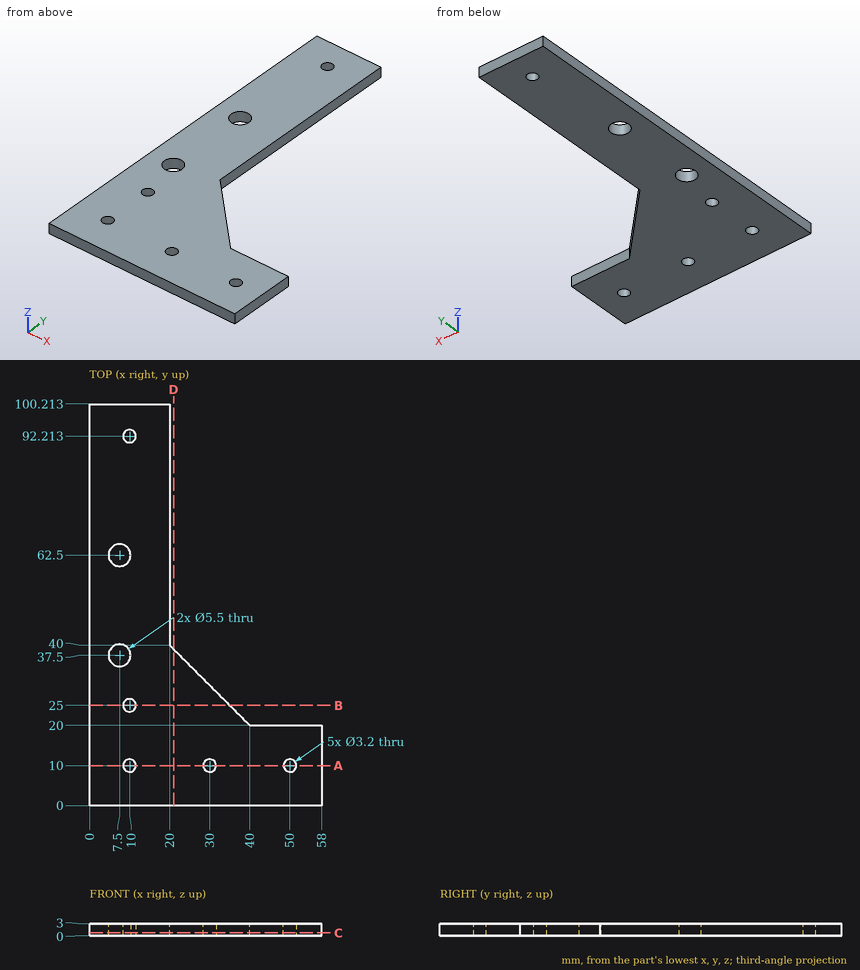
For this review, use the dimensioned drawing (mm, ordinates from the lowest corner) and the shaded views. Coordinates: 2 decimals unless noted, no trailing zeros. Order: outer loops, then holes, each group sorted by start corner. A loop starts at its lowest first (then second) coordinate and runs counter-clockwise, first axis right, second up. Notation, with made-up numbers: M 21,-33.5 L 70,-33.5 A24 ccw 70,4.5 Z; hole C 2.25,-16.75 d11. An arc over 180 degrees is marked long. Answer as a JSON object with one key per item and string values. Group by question number.
1) Wall thickness on L1, parallel to Y at x = 7.5, z = 1.8; L2, parallel to X at y = 75, z = 2.05; L3, parallel to X at y = 35, z = 2.4 (1 decimal): over which ranges is each line inside the solid? List them lowest first.
2) Add section B-B, the plane y = 25. Write out the cut boundary in (x, z).
3) Add section D-D, the plane x = 21. Write out the cut boundary in (y, z), then the cut area to 3 significant figures.
4) Add section A-A, the plane y = 10. Write out the cut boundary in (x, z), then the cut area to 3 significant figures.
5) For pin 1 (1.5 mm diameter, centred on y = 82, z = 1, fed in from +X); pin 2 (1.5 mm diameter, centred on x = 28.5, z = 1.5, fed in from +Y), all flat-tipped, find the tip position at first contact; note any pin that passes through.
6) Add section C-C, the plane z = 0.7. Write out the cut boundary in (x, y).
Computed values:
{
 "1": {"L1": "y = 0 to 34.75, 40.25 to 59.75, 65.25 to 100.21", "L2": "x = 0 to 20", "L3": "x = 0 to 6.4, 8.6 to 25"},
 "2": {"outline": "M 0,0 L 8.4,0 L 8.4,3 L 0,3 Z; M 11.6,0 L 35,0 L 35,3 L 11.6,3 Z"},
 "3": {"outline": "M 0,0 L 39,0 L 39,3 L 0,3 Z", "area": "117 mm^2"},
 "4": {"outline": "M 0,0 L 8.4,0 L 8.4,3 L 0,3 Z; M 11.6,0 L 28.4,0 L 28.4,3 L 11.6,3 Z; M 31.6,0 L 48.4,0 L 48.4,3 L 31.6,3 Z; M 51.6,0 L 58,0 L 58,3 L 51.6,3 Z", "area": "145 mm^2"},
 "5": {"pin 1": "stops at x = 20", "pin 2": "stops at y = 32.25"},
 "6": {"outline": "M 0,0 L 58,0 L 58,20 L 40,20 L 20,40 L 20,100.21 L 0,100.21 Z; hole C 7.5,37.5 d5.5; hole C 7.5,62.5 d5.5; hole C 10,10 d3.2; hole C 10,25 d3.2; hole C 10,92.21 d3.2; hole C 30,10 d3.2; hole C 50,10 d3.2"}
}
